For this review, take the finished solid that the model builds, in its own axes (mm). Give positions to 0.01 mm unless a question says otherwise; leave off trailing zeros. Write each loop counter-clockwise with the first axis right and the second up, starting at its lowest first coordinate (ties: lowest second). Pieces come first, ordered by that corner, then holes.
from build123d import *

# Parameters (mm, degrees)
SKETCH_R   = 53
SKETCH_R_2 = 45
SKETCH_R_3 = 2.5
PAD_DEPTH  = 0.5


with BuildPart() as part:
    # Sketch → Pad (new body)
    with BuildSketch(Plane.XY):
        Circle(SKETCH_R)
        Circle(SKETCH_R_2, mode=Mode.SUBTRACT)
        with Locations((31.496593, 37.536178)):
            Circle(SKETCH_R_3, mode=Mode.SUBTRACT)
        with Locations((48.25558, 8.508761)):
            Circle(SKETCH_R_3, mode=Mode.SUBTRACT)
        with Locations((42.435245, -24.5)):
            Circle(SKETCH_R_3, mode=Mode.SUBTRACT)
        with Locations((16.758987, -46.044938)):
            Circle(SKETCH_R_3, mode=Mode.SUBTRACT)
        with Locations((-16.758987, -46.044938)):
            Circle(SKETCH_R_3, mode=Mode.SUBTRACT)
        with Locations((-42.435245, -24.5)):
            Circle(SKETCH_R_3, mode=Mode.SUBTRACT)
        with Locations((-48.25558, 8.508761)):
            Circle(SKETCH_R_3, mode=Mode.SUBTRACT)
        with Locations((-31.496593, 37.536178)):
            Circle(SKETCH_R_3, mode=Mode.SUBTRACT)
        with Locations((0, 49)):
            Circle(SKETCH_R_3, mode=Mode.SUBTRACT)
    extrude(amount=PAD_DEPTH)


solid = part.part
(1) The part is to be moulded in two halves that separate along X. For faces 1 (the cylindrical face through (-14.45, -47, 0.25)), 2 (the cylindrical face through (28.49, 44.69, 0.25)), 3 (the cylindrical face through (-0.54, 46.56, 0.25)), 4 (the flat face through (-36, 28, 0)), say which applies: +X half, -X half, draft (parallel to the pull), parting line (faces both ways), or undercut.
(2) We need section A-A (x = 0). Write out the cut boundary in (y, z), and give its area (3 significant figures).
(3) We need section C-C (z = 0.15). Count the separate pieces of the cut face and the enclosed holes in it, and give its area (3 significant figures).
(4) For L1, parallel to Y at x = 0, z = 0.3; L2, parallel to X at y = 10, z = 0.1; L3, parallel to Y at x = -19, z = 0.2, list the stretches that pass through material, from the lowest coordinate up.
(5) We need section D-D (x = 20.5). Write out the cut boundary in (y, z).
(6) We need section B-B (y = -20). Write out the cut boundary in (x, z), and give its area (3 significant figures).
The answers:
1. face 1: undercut
1. face 2: parting line
1. face 3: undercut
1. face 4: draft
2. outline: (-53, 0) - (-45, 0) - (-45, 0.5) - (-53, 0.5) - close; (45, 0) - (46.5, 0) - (46.5, 0.5) - (45, 0.5) - close; (51.5, 0) - (53, 0) - (53, 0.5) - (51.5, 0.5) - close
2. area: 5.50 mm2
3. separate pieces: 1
3. enclosed holes: 10
3. area: 2,290 mm2
4. L1: y = -53 to -45, 45 to 46.5, 51.5 to 53
4. L2: x = -52.05 to -50.26, -46.25 to -43.87, 43.87 to 46.25, 50.26 to 52.05
4. L3: y = -49.48 to -47.15, -44.94 to -40.79, 40.79 to 49.48
5. outline: (-48.87, 0) - (-40.06, 0) - (-40.06, 0.5) - (-48.87, 0.5) - close; (40.06, 0) - (48.87, 0) - (48.87, 0.5) - (40.06, 0.5) - close
6. outline: (-49.08, 0) - (-40.31, 0) - (-40.31, 0.5) - (-49.08, 0.5) - close; (40.31, 0) - (49.08, 0) - (49.08, 0.5) - (40.31, 0.5) - close
6. area: 8.77 mm2
